Check sheet for the modelled part. Datum: model origin and axes. Units: mm. A direction names the side the tool comes from. Coordinates: 2 decimals unless noted, no trailing zeros. Write each loop counter-clockwise with the first axis right and the second up, starting at its lowest first coordinate (ties: lowest second). Pieces come first, ordered by that corner, then holes. Notation, with made-up numbers: (37, 49) -> (79, 49) arc R19 cw to (79, 77) -> close; hole circle Ø10 at (30.25, 0.5). An arc over 180 degrees is marked (long way). Put each result on its own line as item: value.
```python
from build123d import *

# Parameters (mm, degrees)
F1_DEPTH = 44.45


with BuildPart() as f1:
    # F0 (on Top) → F1 (new body)
    with BuildSketch(Plane.XY):
        with BuildLine():
            Line((38.1, 0), (0, 0))
            Line((0, 0), (0, 38.1))
            Line((0, 38.1), (3.175, 38.1))
            Line((3.175, 38.1), (0, 41.275))
            ThreePointArc((0, 41.275), (-2.245064, 40.345064), (-3.175, 38.1))
            Line((-3.175, 38.1), (-3.175, 0))
            ThreePointArc((-3.175, 0), (-2.245064, -2.245064), (0, -3.175))
            Line((0, -3.175), (38.1, -3.175))
            Line((38.1, -3.175), (38.1, -22.225))
            Line((38.1, -22.225), (-3.175, -22.225))
            Line((-3.175, -22.225), (-3.175, -25.4))
            Line((-3.175, -25.4), (38.1, -25.4))
            ThreePointArc((38.1, -25.4), (40.345064, -24.470064), (41.275, -22.225))
            Line((41.275, -22.225), (41.275, -3.175))
            Line((41.275, -3.175), (41.275, 38.1))
            ThreePointArc((41.275, 38.1), (40.345064, 40.345064), (38.1, 41.275))
            Line((38.1, 41.275), (34.925, 38.1))
            Line((34.925, 38.1), (38.1, 38.1))
            Line((38.1, 38.1), (38.1, 0))
        make_face()
    extrude(amount=F1_DEPTH)


solid = f1.part
```
Q1. Depth check by flat-ended pin: P1, Ø1, axis at x = 1.5, z = 14.5, coming from the +Y side (3 decimals); P2, Ø5.5, axis at y = -11, z = 32.5, coming from the -X side. Enter the tip coordinate at first touch or a pass-through.
Recorded:
P1: stops at y = 40.275
P2: stops at x = 38.1
Q2. Cross-section at B-B (x = 18.5). Record the cut outline in (y, z) (3 decimals).
Recorded:
outline: (-25.4, 0) -> (-22.225, 0) -> (-22.225, 44.45) -> (-25.4, 44.45) -> close; (-3.175, 0) -> (0, 0) -> (0, 44.45) -> (-3.175, 44.45) -> close
Q3. Mould release check, pull along X, two halves, no side actions. Record for faces 5 (the flat face through (41.275, 8, 22)), 6 (the flat face through (36.535, 39.71, 21.914)), 7 (the flat face through (21, -2, 44.45)): released by +X, released by -X, zero draft, split by the parting line, or undercut.
Recorded:
face 5: released by +X
face 6: undercut
face 7: zero draft
Q4. Cross-section at C-C (z = 12.5). Record the cut outline in (x, y) (3 decimals).
Recorded:
outline: (-3.175, -25.4) -> (38.1, -25.4) arc R3.175 ccw to (41.275, -22.225) -> (41.275, 38.1) arc R3.175 ccw to (38.1, 41.275) -> (34.925, 38.1) -> (38.1, 38.1) -> (38.1, 0) -> (0, 0) -> (0, 38.1) -> (3.175, 38.1) -> (0, 41.275) arc R3.175 ccw to (-3.175, 38.1) -> (-3.175, 0) arc R3.175 ccw to (0, -3.175) -> (38.1, -3.175) -> (38.1, -22.225) -> (-3.175, -22.225) -> close
Q5. Cross-section at D-D (x = 37). Record the cut outline in (y, z) (3 decimals), plus the area to 3 significant figures.
Recorded:
outline: (-25.4, 0) -> (-22.225, 0) -> (-22.225, 44.45) -> (-25.4, 44.45) -> close; (-3.175, 0) -> (0, 0) -> (0, 44.45) -> (-3.175, 44.45) -> close; (38.1, 0) -> (40.175, 0) -> (40.175, 44.45) -> (38.1, 44.45) -> close
area: 374 mm2
Q6. Material ranges on line 1 along Y through (x, z) = (14, 14) (3 decimals); line 2 along X through (y, z) = (25, 30.5) (3 decimals); line 3 along Y through (x, z) = (2.5, 42) (3 decimals), recorded low to high.
Recorded:
line 1: y = -25.4 to -22.225, -3.175 to 0
line 2: x = -3.175 to 0, 38.1 to 41.275
line 3: y = -25.4 to -22.225, -3.175 to 0, 38.1 to 38.775
Q7. Tool access check on faces 1 (the flat face through (17, -25.4, 22)), 2 (the flat face through (1.61, 39.665, 21.914)), 3 (the cylindrical face through (-2.27, -2.22, 21.91)), 4 (the flat face through (19, 0, 22)). Record the directions out of +Z, -Z, +X, -X, +Y, -Y that give a thin tool (end or side, any length) a straight path to the whole face; none if there is none.
Recorded:
face 1: +Z, -Z, +X, -X, -Y
face 2: +Z, -Z, +Y
face 3: +Z, -Z, -X
face 4: +Z, -Z
Q8. Cross-section at A-A (y = 33). Record the cut outline in (x, z) (3 decimals), plus the area to 3 significant figures.
Recorded:
outline: (-3.175, 0) -> (0, 0) -> (0, 44.45) -> (-3.175, 44.45) -> close; (38.1, 0) -> (41.275, 0) -> (41.275, 44.45) -> (38.1, 44.45) -> close
area: 282 mm2
